The figure shows three views and two pictorial views of one solid part (mm, origin at its lowest corner). Answer the questions. A direction names the side the tool comes from. Coordinates: 2 decimals unless noted, no trailing zeros. Write each loop counter-clockwise with the first axis right and the second up, starting at its lowest first coordinate (ties: lowest second). Pieces come first, ordered by that corner, then holes. Notation, with made-up numbers: (31.5, 84) - (47.5, 84) arc R14 ccw to (47.5, 97) - close; hole circle Ø10 at (31.5, 51). An arc over 180 degrees is marked (long way). Use a Markdown table: item, result. Add a question column.
(1) The part is cut by section D-D, the plane z = 2. Give the vertices of the cut face in (x, y).
(2) The part is cut by section A-A, the plane y = 10. Give the vertices of the cut face in (x, z) (1 decimal).
(3) For a pull along X with two mould halves and no side action, classify the marked faces 1, 2, 3 and 4 as released by +X, released by -X, zero draft, split by the parting line, or undercut.
(4) Find the intervals of material crossed by line 1 (X direction, y = 31, z = 6); line 2 (Z direction, x = 30, y = 34.25); line 3 (X direction, y = 2, z = 6), in increasing order. Write a range as from..to.
(5) The part is cut by section C-C, the plane x = 30.5. Give the vertices of the cut face in (y, z) (1 decimal).
(6) A tool of negligible diameter and unlimited length cuts with its end or side. For the marked faces 5 and 6, from which of +Z, -Z, +X, -X, +Y, -Y can it reach the whole face along a straight path? Write none if from no direction.
(7) The part is cut by section B-B, the plane z = 4.5. Give the vertices of the cut face in (x, y).
(8) Given pin 1 Ø3.5 at (x, z) = (30, 6) entering from -Y; pin 2 Ø1 at (y, z) = (19, 7.5) entering from -X; pin 3 Ø5 at (y, z) = (23, 10) entering from -X, each flat-ended and moving along its own axis, determine where each tip first touches the part or whether it passes through.
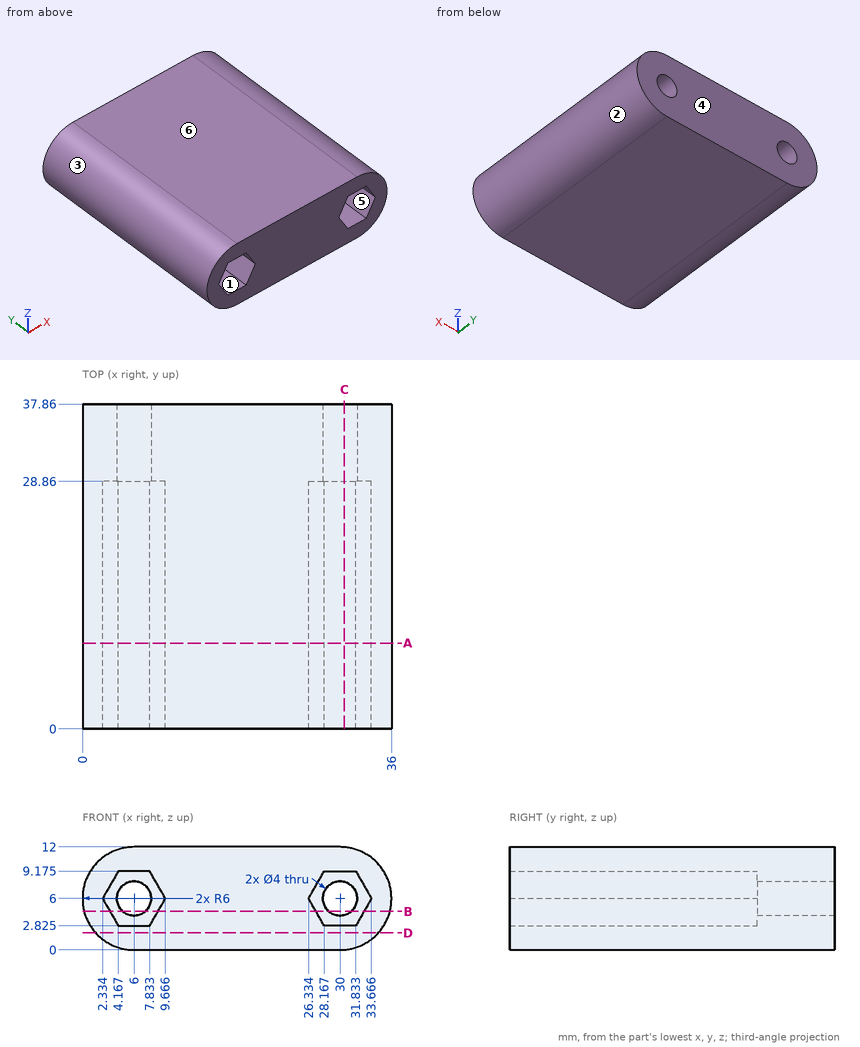
Model answer:
| question | item | result |
|---|---|---|
| 1 | outline | (1.53, 0) - (34.47, 0) - (34.47, 37.86) - (1.53, 37.86) - close |
| 2 | outline | (6, 0) - (30, 0) arc R6 ccw to (30, 12) - (6, 12) arc R6 ccw to start; hole (2.3, 6) - (4.2, 2.8) - (7.8, 2.8) - (9.7, 6) - (7.8, 9.2) - (4.2, 9.2) - close; hole (26.3, 6) - (28.2, 2.8) - (31.8, 2.8) - (33.7, 6) - (31.8, 9.2) - (28.2, 9.2) - close |
| 3 | face 1 | undercut |
| 3 | face 2 | released by +X |
| 3 | face 3 | released by -X |
| 3 | face 4 | zero draft |
| 4 | line 1 | 0..4, 8..28, 32..36 |
| 4 | line 2 | 0..4, 8..12 |
| 4 | line 3 | 0..2.33, 9.67..26.33, 33.67..36 |
| 5 | outline | (0, 0) - (37.9, 0) - (37.9, 4.1) - (28.9, 4.1) - (28.9, 2.8) - (0, 2.8) - close; (0, 9.2) - (28.9, 9.2) - (28.9, 7.9) - (37.9, 7.9) - (37.9, 12) - (0, 12) - close |
| 6 | face 5 | -Y |
| 6 | face 6 | +Z, +X, -X, +Y, -Y |
| 7 | outline | (0.19, 0) - (3.2, 0) - (3.2, 28.86) - (4.68, 28.86) - (4.68, 37.86) - (0.19, 37.86) - close; (7.32, 28.86) - (8.8, 28.86) - (8.8, 0) - (27.2, 0) - (27.2, 28.86) - (28.68, 28.86) - (28.68, 37.86) - (7.32, 37.86) - close; (31.32, 28.86) - (32.8, 28.86) - (32.8, 0) - (35.81, 0) - (35.81, 37.86) - (31.32, 37.86) - close |
| 8 | pin 1 | through |
| 8 | pin 2 | x = 0.08 |
| 8 | pin 3 | x = 0.19 |
